```python
from build123d import *

# Parameters (mm, degrees)
PAD039_DEPTH = 4
PAD040_DEPTH = 20


with BuildPart() as tentingfoot:
    # Sketch060 → Pad039 (new body)
    with BuildSketch(Plane.XZ):
        with BuildLine():
            ThreePointArc((-21.1964126557, -41.8543733369), (-9.7268365797, -41.3536008307), (-1.970721194, -32.889286175))
            Line((-1.970721194, -32.889286175), (10, 0))
            ThreePointArc((19.6984611198, -1.705646413), (15.5645105895, 3.2143243008), (10, 0))
            Line((19.6984611198, -1.705646413), (19.7057836753, -9.9252842627))
            ThreePointArc((19.2233278161, -12.6685722951), (19.5848668778, -11.3180871255), (19.7057836753, -9.9252842627))
            Line((19.2233278161, -12.6685722951), (3.4048800097, -56.129400454))
            Line((-34.1828248217, -42.448594721), (3.4048800097, -56.129400454))
            Line((-32.4727241051, -37.750131617), (-34.1828248217, -42.448594721))
            Line((-21.1964126557, -41.8543733369), (-32.4727241051, -37.750131617))
        make_face()
        with BuildLine():
            ThreePointArc((16.6718176076, -2.4283430176), (15.4167054049, 0.263253787), (12.7251086003, -0.9918584156))
            Line((12.7251086003, -0.9918584156), (6.7397560921, -17.4364792794))
            ThreePointArc((6.7397560921, -17.4364792794), (7.9948682947, -20.128076084), (10.6864650994, -18.8729638814))
            Line((10.6864650994, -18.8729638814), (16.6718176076, -2.4283430176))
        make_face(mode=Mode.SUBTRACT)
        with BuildLine():
            ThreePointArc((7.2662547771, -28.2698888178), (6.0111449398, -25.5782909102), (3.3195470322, -26.8334007475))
            Line((3.3195470322, -26.8334007475), (-2.6658199272, -43.2780163515))
            ThreePointArc((-2.6658199272, -43.2780163515), (-1.4107100899, -45.9696142591), (1.2808878177, -44.7145044217))
            Line((1.2808878177, -44.7145044217), (7.2662547771, -28.2698888178))
        make_face(mode=Mode.SUBTRACT)
    extrude(amount=PAD039_DEPTH)

    # Sketch061 → Pad040 (join)
    with BuildSketch(Plane.XZ):
        Polygon((5.1149807264, -51.4309373501), (-32.4727241051, -37.750131617), (-34.1828248217, -42.448594721), (3.4048800097, -56.129400454), align=None)
    extrude(amount=-PAD040_DEPTH)


with BuildPart() as tentingfoot_1:
    # Body013 placement: moved
    add(tentingfoot.part.moved(Location((140, 55, 0))))


with BuildPart() as part_mirroring001:
    # Part__Mirroring001: instance of TentingFoot
    add(tentingfoot_1.part.mirror(Plane(origin=(133.8426055908, 1.9073e-06, -12.4421358109), x_dir=(1, 0, 0), z_dir=(0, 1, -1.192e-07))))


solid = part_mirroring001.part
```
Verification items for the finished model (mm, model axes). A direction names the side the tool comes from. Round coordinates to 2 decimals unless told otherwise and drop trailing zeros. Write each loop counter-clockwise with the first axis right and the second up, starting at its lowest first coordinate (ties: lowest second). Pieces come first, ordered by that corner, then holes.
1. Access from +Z, -Z, +X, -X, +Y, -Y to the whole of each face (thin tool, end or side, straight path). Record for faces 1 (the flat face through (148, -55, -28)), 2 (the flat face through (140.37, -53.03, -34.94)), 3 (the cylindrical face through (130.123, -53.028, -41.422)).
2. Section check D-D on x = 122.5. Enter the section's corners in (y, z), plus the area to 3 significant figures.
3. Section check A-A on x = 139. Enter the section's corners in (y, z), plus the area to 3 significant figures.
4. Scan lines: L1, parallel to X at y = -52.25, z = -33; L2, parallel to Y at x = 149, z = -7.5; L3, parallel to Z at x = 110, y = -59.5. Record each from-to range of solid material in increasing order.
5. Section check C-C on y = -66.5. Enter the section's corners in (x, z).
6. Draft check along X on faces 4 (the cylindrical face through (146.054, -53.028, -25.595)), 5 (the flat face through (141, -51, -31)), 6 (the flat face through (143.931, -53.028, -16.675)). Enter one of: +X half, -X half, draft (parallel to the pull), parting line (faces both ways), or undercut.
7. Section check B-B on z = -30. Enter the section's corners in (x, y).
8. Gauge pin test, flat ends, axial feed: P1, Ø5, axis at x = 145.5, z = -46, coming from the -Y side; P2, Ø12, axis at x = 144.5, z = -32, coming from the +Y side. Record the tip position at first contact, or that the pin passes through.
Answer:
1. face 1: +Z, +X, -Y
1. face 2: +Y, -Y
1. face 3: +Z, +Y, -Y
2. outline: (-75, -48.52) - (-51, -48.52) - (-51, -42.69) - (-55, -42.69) - (-55, -43.2) - (-75, -43.2) - close
2. area: 130 mm2
3. outline: (-75, -54.53) - (-51, -54.53) - (-51, -46.07) - (-55, -46.07) - (-55, -49.21) - (-75, -49.21) - close; (-55, -38.7) - (-51, -38.7) - (-51, -30.22) - (-55, -30.22) - close
3. area: 174 mm2
4. L1: x = 137.99 to 141.08, 145.54 to 151.82
4. L2: y = -55 to -51
4. L3: z = -43.97 to -38.65
5. outline: (105.82, -42.45) - (143.4, -56.13) - (145.11, -51.43) - (107.53, -37.75) - close
6. face 4: undercut
6. face 5: draft
6. face 6: -X half
7. outline: (139.08, -55) - (142.17, -55) - (142.17, -51) - (139.08, -51) - close; (146.64, -55) - (152.92, -55) - (152.92, -51) - (146.64, -51) - close
8. P1: stops at y = -55
8. P2: stops at y = -51
